from build123d import *

# Parameters (mm, degrees)
BOSS_EXTRU_1_DEPTH = 40
CONG_1_R           = 2
COQUE1_START       = 4
COQUE1_DEPTH       = 32


# Read off the part's stored shape, not the designer's step: Coque1
with BuildPart() as part:
    # Esquisse1 → Boss.-Extru.1 (new body)
    with BuildSketch(Plane.XY):
        Polygon((0, 0), (0, 400), (-350, 400), (-350, 360), (-40, 0), align=None)
        Polygon((-297.798149171, 360), (-40, 360), (-40, 60.621504188), align=None, mode=Mode.SUBTRACT)
    extrude(amount=BOSS_EXTRU_1_DEPTH)

    # Congé1
    cong_1_edges = [part.edges().sort_by_distance(p)[0] for p in [
        (-175, 400, 40),
        (-350, 380, 40),
        (-195, 180, 40),
        (-168.899074586, 210.310752094, 0),
        (-40, 210.310752094, 0),
        (-168.899074586, 360, 0),
        (-168.899074586, 210.310752094, 40),
        (-40, 210.310752094, 40),
        (-168.899074586, 360, 40),
        (-20, 0, 40),
        (-195, 180, 0),
        (-350, 380, 0),
        (-175, 400, 0),
        (0, 200, 0),
        (-20, 0, 0),
        (0, 200, 40),
    ]]
    fillet(cong_1_edges, radius=CONG_1_R)

    # Coque1 outline → Coque1 (cut)
    with BuildSketch(Plane.XY.offset(COQUE1_START)):
        Polygon((-38.165789547, 4), (-4, 4), (-4, 396), (-346, 396), (-346, 361.484889559), align=None)
        Polygon((-36, 364), (-36, 49.846292049), (-306.521248514, 364), align=None, mode=Mode.SUBTRACT)
    extrude(amount=COQUE1_DEPTH, mode=Mode.SUBTRACT)


solid = part.part
Geometry: final body of the model. Coordinates: model frame, mm. A direction names the side the tool comes from. Coordinates: 2 decimals unless noted, no trailing zeros. Loops run counter-clockwise (first coordinate to the right, second up) from the corner with the lowest first, then second, coordinate; pieces in that order, holes last. Notation, with made-up numbers: (-4.5, 7.5) - (43.5, 7.5) arc R17 ccw to (43.5, 31.5) - close; hole circle Ø2 at (17, 80). An arc over 180 degrees is marked (long way). Put each result on its own line as item: value. Start each with the question number.
Q1. Line query: line 1 (X direction, y = 65.5, z = 31.5); line 2 (X direction, y = 267, z = 12.5); line 3 (X direction, y = 55.5, z = 29.5). Output: solid intervals per line, ascending.
Q2. Cut plane B-B, the plane y = 324.5. Give the number of separate pieces and of enclosed holes in the cut face, and give its area (3 significant figures).
Q3. Set-up query: faces 1 (the flat face through (-171, 360, 20)), 2 (the flat face through (-173, 396, 20)), 3 (the flat face through (-350, 380, 20)). Return all of +Z, -Z, +X, -X, +Y, -Y with unobstructed straight access to the full face (end or side cutting, diameter ignored); none if empty.
Q4. Pull-direction query (Z, two-part tool) for faces 4 (the cylindrical face through (-170.85, 211.7, 39.4)), 5 (the flat face through (-20, 0, 20)), 6 (the flat face through (-176, 201, 36)); classes: released by +Z, released by -Z, zero draft, split by the parting line, or undercut.
Q5. Pin query (flat end, axial travel): pin 1 Ø3 at (y, z) = (345, 9) entering from +X; pin 2 Ø16 at (x, z) = (-133.5, 26) entering from -Y; pin 3 Ø18 at (x, z) = (-139, 28) entering from -Y; pin 4 Ø2 at (x, z) = (-219, 20.5) entering from -Y. Return the tip coordinate at first contact, or that it passes through.
Q6. Cut plane A-A, the plane z = 20. Return loops of the section in (x, y).
Filled sheet:
1. line 1: -96.4 to -91.12, -49.48 to -44.2, -40 to -36, -4 to 0
1. line 2: -269.92 to -264.64, -222.99 to -217.71, -40 to -36, -4 to 0
1. line 3: -87.79 to -82.51, -40.87 to -36, -4 to 0
2. separate pieces: 2
2. enclosed holes: 2
2. area: 1,320 mm²
3. face 1: +Z, -Z
3. face 2: none
3. face 3: +Z, -Z, -X, +Y, -Y
4. face 4: released by +Z
4. face 5: zero draft
4. face 6: undercut
5. pin 1: x = 0
5. pin 2: y = 99.29
5. pin 3: y = 104.52
5. pin 4: y = 206.71
6. outline: (-350, 360) - (-40, 0) - (0, 0) - (0, 400) - (-350, 400) - close; (-306.52, 364) - (-36, 49.85) - (-36, 364) - close; hole (-346, 361.48) - (-38.17, 4) - (-4, 4) - (-4, 396) - (-346, 396) - close; hole (-297.8, 360) - (-40, 60.62) - (-40, 360) - close
